```python
from build123d import *

# Parameters (mm, degrees)
BOSS_EXTRUDE1_DEPTH = 48
SKETCH3_R           = 4.1
CUT_EXTRUDE1_DEPTH  = 41.7
SKETCH4_R           = 3.15
CUT_EXTRUDE2_DEPTH  = 4.7
SKETCH5_R           = 4.1
SKETCH5_R_2         = 2.1
BOSS_EXTRUDE2_DEPTH = 3


with BuildPart() as part:
    # Sketch2 → Boss-Extrude1 (new body)
    with BuildSketch(Plane(origin=(0, 0, 0), x_dir=(1, 0, 0), z_dir=(0, 1, 0))):
        Polygon((0, 0), (0, -20), (0, -48), (34.641016151, -48), (34.641016151, -20), align=None)
    extrude(amount=BOSS_EXTRUDE1_DEPTH)

    # Sketch3 → Cut-Extrude1 (cut)
    with BuildSketch(Plane(origin=(0, 0, 0), x_dir=(-0.8660254037844417, 0, -0.4999999999999947), z_dir=(0.49999999999999484, 0, -0.8660254037844418))):
        with Locations((-7, 40)):
            Circle(SKETCH3_R)
        with Locations((-7, 8)):
            Circle(SKETCH3_R)
    extrude(amount=-CUT_EXTRUDE1_DEPTH, mode=Mode.SUBTRACT)

    # Sketch4 → Cut-Extrude2 (cut)
    with BuildSketch(Plane.XY.offset(48)):
        with Locations((8.641016151, 40)):
            Circle(SKETCH4_R)
        with Locations((24.641016151, 40)):
            Circle(SKETCH4_R)
        with Locations((8.641016151, 8)):
            Circle(SKETCH4_R)
        with Locations((24.641016151, 8)):
            Circle(SKETCH4_R)
    extrude(amount=-CUT_EXTRUDE2_DEPTH, mode=Mode.SUBTRACT)

    # Sketch5 → Boss-Extrude2 (add)
    # profile 1 of 2: a face of its own
    with BuildSketch(Plane(origin=(0, 0, 0), x_dir=(-0.8660254037844417, 0, -0.4999999999999947), z_dir=(0.49999999999999484, 0, -0.8660254037844418))):
        with Locations((-7, 40)):
            Circle(SKETCH5_R)
        with Locations((-7, 40)):
            Circle(SKETCH5_R_2, mode=Mode.SUBTRACT)
    # profile 2 of 2: a face of its own
    with BuildSketch(Plane(origin=(0, 0, 0), x_dir=(-0.8660254037844417, 0, -0.4999999999999947), z_dir=(0.49999999999999484, 0, -0.8660254037844418))):
        with Locations((-7, 8)):
            Circle(SKETCH5_R)
        with Locations((-7, 8)):
            Circle(SKETCH5_R_2, mode=Mode.SUBTRACT)
    extrude(amount=-BOSS_EXTRUDE2_DEPTH)


solid = part.part
```
Source: CAD feature listing. Evaluate the final solid. Frame: model axes, mm. A direction names the side the tool comes from. Round coordinates to 2 decimals unless told otherwise and drop trailing zeros. Order: outer loops, then holes, each group sorted by start corner. A loop starts at its lowest first (then second) coordinate and runs counter-clockwise, first axis right, second up. Notation, with made-up numbers: (38.5, 86.5) -> (67.5, 86.5) arc R26 cw to (67.5, 114.5) -> close; hole circle Ø11 at (25.25, 40). An arc over 180 degrees is marked (long way). Use CSV: the item, a comma, the result in double quotes.
(1) First-contact query: pin 1 Ø1 at (x, y) = (20, 36.5) entering from -Z; pin 2 Ø1 at (x, y) = (23.5, 35) entering from -Z; pin 3 Ø7 at (x, y) = (8.64, 8) entering from -Z. Flat tips, straight axial feed; report the tip coordinate or a pass-through.
Report:
pin 1,"z = 11.26"
pin 2,"z = 13.28"
pin 3,"z = 3.36"
(2) Ray query, L1, parallel to Y at x = 4, z = 6.5; L2, parallel to Y at x = 5.5, z = 5; L3, parallel to Z at x = 7, y = 11.5. Return the intervals inside material, ascending.
Report:
L1,"0 to 3.91, 12.09 to 35.91, 44.09 to 48"
L2,"0 to 5.92, 10.08 to 37.92, 42.08 to 48"
L3,"4.04 to 48"
(3) Access query for faces 4 (the face through (3.034, 6.235, 5.216)), 5 (the face through (9, 8, 43.3)), 6 (the face through (17, 24, 48)). Directions: +Z, -Z, +X, -X, +Y, -Y. A direction counts if a zero-diameter tool reaches every point of the face in a straight line with its end or side. Return the directions, or none.
Report:
face 4,"none"
face 5,"+Z"
face 6,"+Z, +X, -X, +Y, -Y"
(4) Section D-D on y = 22. Return the cut outline in (x, z).
Report:
outline,"(0, 0) -> (34.64, 20) -> (34.64, 48) -> (0, 48) -> close"
(5) Pull-direction query (Z, two-part tool) for faces 1 (the face through (5.56, 10.08, 4.92)), 2 (the face through (9, 40, 43.3)), 3 (the face through (23.958, 36.925, 45.683)); classes: +Z half, -Z half, draft (parallel to the pull), parting line (faces both ways), or undercut.
Report:
face 1,"undercut"
face 2,"+Z half"
face 3,"draft"
(6) Section B-B on x = 11. Return the cut outline in (y, z), and give its area (3 significant figures).
Report:
outline,"(0, 6.35) -> (48, 6.35) -> (48, 48) -> (42.09, 48) -> (42.09, 43.3) -> (37.91, 43.3) -> (37.91, 48) -> (10.09, 48) -> (10.09, 43.3) -> (5.91, 43.3) -> (5.91, 48) -> (0, 48) -> close"
area,"1,960 mm^2"
(7) Section C-C on x = 7. Count the separate pieces of the cut face and the enclosed holes in it, and give its area (3 significant figures).
Report:
separate pieces,"1"
enclosed holes,"2"
area,"2,030 mm^2"
(8) Section A-A on y = 40. Return the cut outline in (x, z), and give its area (3 significant figures).
Report:
outline,"(0, 0) -> (4.24, 2.45) -> (2.74, 5.05) -> (1.01, 4.05) -> (0, 5.8) -> close; (0, 22.2) -> (8.11, 8.15) -> (6.38, 7.15) -> (7.88, 4.55) -> (34.64, 20) -> (34.64, 48) -> (27.79, 48) -> (27.79, 43.3) -> (21.49, 43.3) -> (21.49, 48) -> (11.79, 48) -> (11.79, 43.3) -> (5.49, 43.3) -> (5.49, 48) -> (0, 48) -> close"
area,"1,170 mm^2"
